Build history of the part. All positions in model axes, mm. A direction names the side the tool comes from. Round coordinates to 2 decimals unless told otherwise and drop trailing zeros. Loops run counter-clockwise (first coordinate to the right, second up) from the corner with the lowest first, then second, coordinate; pieces in that order, holes last.
from build123d import *

# Parameters (mm, degrees)
BOSS_EXTRUDE1_DEPTH = 18.5
SKETCH3_W           = 10
SKETCH3_H           = 10
BOSS_EXTRUDE2_DEPTH = 3
SKETCH5_R           = 1.375
CUT_EXTRUDE1_DEPTH  = 3


with BuildPart() as part:
    # Sketch1 → Boss-Extrude1 (new body)
    with BuildSketch(Plane(origin=(0, 0, 0), x_dir=(1, 0, 0), z_dir=(0, 1, 0))):
        Polygon((-34, 0), (-37.608439182, 6.25), (-34, 6.25), (-34, 12), (-15.5, 12), (-15.5, 6.25), (15.5, 6.25), (15.5, 12), (34, 12), (34, 6.25), (37.608439182, 6.25), (34, 0), align=None)
    extrude(amount=BOSS_EXTRUDE1_DEPTH)

    # Sketch2 → Cut-Revolve1 (revolve, cut)
    with BuildSketch(Plane(origin=(0, 9.25, 0), x_dir=(1, 0, 0), z_dir=(0, 1, 0))):
        with BuildLine():
            Line((-24.75, 12), (-24.75, 0))
            Line((-24.75, 0), (-31.75, 0))
            ThreePointArc((-31.75, 0), (-31.297900427, 2.474873734), (-30, 4.630064794))
            Line((-30, 4.630064794), (-30, 12))
            Line((-30, 12), (-24.75, 12))
        make_face()
    cut_revolve1 = revolve(axis=Axis((-24.75, 9.25, -35.715820775), (0, 0, 1)), mode=Mode.SUBTRACT)

    # Mirror1: Cut-Revolve1 across plane
    add(cut_revolve1.mirror(Plane(origin=(0, 0, 0), x_dir=(0, 0, 1), z_dir=(1, 0, 0))), mode=Mode.SUBTRACT)

    # Sketch3 → Boss-Extrude2 (add)
    with BuildSketch(Plane(origin=(0, 0, 0), x_dir=(1, 0, 0), z_dir=(0, 1, 0))):
        with Locations((-29, 17)):
            Rectangle(SKETCH3_W, SKETCH3_H)
        with Locations((29, 17)):
            Rectangle(SKETCH3_W, SKETCH3_H)
    extrude(amount=BOSS_EXTRUDE2_DEPTH)

    # Sketch5 → Cut-Extrude1 (cut)
    with BuildSketch(Plane(origin=(0, 3, 0), x_dir=(1, 0, 0), z_dir=(0, 1, 0))):
        with Locations((-29, 17)):
            Circle(SKETCH5_R)
    cut_extrude1 = extrude(amount=-CUT_EXTRUDE1_DEPTH, mode=Mode.SUBTRACT)

    # Mirror2: Cut-Extrude1 across plane
    add(cut_extrude1.mirror(Plane(origin=(0, 0, 0), x_dir=(0, 0, 1), z_dir=(1, 0, 0))), mode=Mode.SUBTRACT)


solid = part.part
(1) Slice it at A-A on z = -7. List the corners of the cut face in (x, y).
Responses:
outline: (-34, 0) - (-15.5, 0) - (-15.5, 18.5) - (-34, 18.5) - close; (15.5, 0) - (34, 0) - (34, 18.5) - (15.5, 18.5) - close; hole circle Ø10.5 at (-24.75, 9.25); hole circle Ø10.5 at (24.75, 9.25)
(2) Slice it at C-C on y = 9.25. List the corners of the cut face in (x, z), plus the area to 3 significant figures.
Responses:
outline: (-37.61, -6.25) - (-34, -6.25) - (-34, -12) - (-30, -12) - (-30, -4.63) arc R7 cw to (-31.75, 0) - (-34, 0) - close; (-19.5, -12) - (-15.5, -12) - (-15.5, -6.25) - (15.5, -6.25) - (15.5, -12) - (19.5, -12) - (19.5, -4.63) arc R7 cw to (17.75, 0) - (-17.75, 0) arc R7 cw to (-19.5, -4.63) - close; (30, -12) - (34, -12) - (34, -6.25) - (37.61, -6.25) - (34, 0) - (31.75, 0) arc R7 cw to (30, -4.63) - close
area: 386 mm2
(3) Pin check, flat tips, straight feed: P1, Ø3, axis at x = 28.5, y = 7.5, coming from the +Z side; P2, Ø4.5, axis at x = 29, z = -17, coming from the +Y side; P3, Ø9, axis at x = 26.5, y = 10, coming from the -Z side. Stop position of each tip, or through.
Responses:
P1: stops at z = -4.15
P2: stops at y = 3
P3: stops at z = -12
(4) Slice it at B-B on z = -13.5. List the corners of the cut face in (x, y).
Responses:
outline: (-34, 0) - (-24, 0) - (-24, 3) - (-34, 3) - close; (24, 0) - (34, 0) - (34, 3) - (24, 3) - close
(5) Which spindle directions (+Z, -Z, +X, -X, +Y, -Y) get a long thin tool onto all of the face, cutting with end or side? Do faces 4 (the face through (34, 7, -11)), 5 (the face through (-34, 7, -11)), 6 (the face through (35.83, 9.12, -3.17)), 7 (the face through (15.5, 9, -9)), 8 (the face through (-28, 3, -18.2)). Say none if no direction does.
Responses:
face 4: -Z, +X, +Y, -Y
face 5: -Z, -X, +Y, -Y
face 6: +Z, +X, +Y, -Y
face 7: -Z, +Y, -Y
face 8: -Z, +X, -X, +Y
(6) Probe line 1 (X direction, y = 2.1, z = -17) (3 decimals); line 2 (X direction, y = 9.25, z = -9.25); line 3 (Z direction, x = -29, y = 0.8) (3 decimals). List the from-to ranges inside material, lowest first.
Responses:
line 1: x = -34 to -30.375, -27.625 to -24, 24 to 27.625, 30.375 to 34
line 2: x = -34 to -30, -19.5 to -15.5, 15.5 to 19.5, 30 to 34
line 3: z = -22 to -18.375, -15.625 to 0
(7) Slice it at D-D on z = -17. List the corners of the cut face in (x, y) (3 decimals), plus the area to 3 significant figures.
Responses:
outline: (-34, 0) - (-30.375, 0) - (-30.375, 3) - (-34, 3) - close; (-27.625, 0) - (-24, 0) - (-24, 3) - (-27.625, 3) - close; (24, 0) - (27.625, 0) - (27.625, 3) - (24, 3) - close; (30.375, 0) - (34, 0) - (34, 3) - (30.375, 3) - close
area: 43.5 mm2
(8) Pull direction Y, two halves, no side cores. Call faces 1 (the face through (1, 18.5, -6)), 2 (the face through (-19.505, 9.019, -8.367)), 3 (the face through (20.5, 13.2, -12)): +Y half, -Y half, draft (parallel to the pull), parting line (faces both ways), or undercut.
Responses:
face 1: +Y half
face 2: undercut
face 3: draft
